Verification items for the finished model (mm, model axes). A direction names the side the tool comes from. Coordinates: 2 decimals unless noted, no trailing zeros. Order: outer loops, then holes, each group sorted by start corner. A loop starts at its lowest first (then second) coordinate and runs counter-clockwise, first axis right, second up. Notation, with made-up numbers: (57, 53.25) -> (102, 53.25) arc R17 cw to (102, 84.25) -> close; hole circle Ø9 at (84, 41). An arc over 180 degrees is marked (long way). Answer as CSV lines item,"result".
```python
from build123d import *

# Parameters (mm, degrees)
SKETCH_1_W          = 40
SKETCH_1_H          = 40
SKETCH_1_W_2        = 38
SKETCH_1_H_2        = 38
EXTRUDE_1_DEPTH     = 160
SKETCH_2_R          = 2.1
CUT_EXTRUDE_1_DEPTH = 170.705627485
SKETCH_4_R          = 2.1
CUT_EXTRUDE_2_DEPTH = 170.705627485


with BuildPart() as part:
    # 草图1 → 凸台-拉伸1 (new body)
    with BuildSketch(Plane.XY):
        with Locations((20, 20)):
            Rectangle(SKETCH_1_W, SKETCH_1_H)
        with Locations((20, 20)):
            Rectangle(SKETCH_1_W_2, SKETCH_1_H_2, mode=Mode.SUBTRACT)
    extrude(amount=EXTRUDE_1_DEPTH)

    # 草图2 → 切除-拉伸1 (cut, through all)
    with BuildSketch(Plane.XZ):
        with Locations(Location((8, 6, 0), (0, 0, 270))):
            Circle(SKETCH_2_R)
        with Locations(Location((32, 22, 0), (0, 0, 270))):
            Circle(SKETCH_2_R)
        with Locations(Location((8, 22, 0), (0, 0, 270))):
            Circle(SKETCH_2_R)
        with Locations(Location((32, 6, 0), (0, 0, 270))):
            Circle(SKETCH_2_R)
    extrude(amount=-CUT_EXTRUDE_1_DEPTH, mode=Mode.SUBTRACT)

    # 草图4 → 切除-拉伸2 (cut, through all)
    with BuildSketch(Plane.ZY):
        with Locations((138, 10)):
            Circle(SKETCH_4_R)
        with Locations((153, 30)):
            Circle(SKETCH_4_R)
        with Locations((153, 10)):
            Circle(SKETCH_4_R)
        with Locations((138, 30)):
            Circle(SKETCH_4_R)
        with Locations((83, 23)):
            Circle(SKETCH_4_R)
        with Locations((65, 7)):
            Circle(SKETCH_4_R)
        with Locations((65, 23)):
            Circle(SKETCH_4_R)
        with Locations((47, 7)):
            Circle(SKETCH_4_R)
        with Locations((47, 23)):
            Circle(SKETCH_4_R)
        with Locations((83, 7)):
            Circle(SKETCH_4_R)
    extrude(amount=-CUT_EXTRUDE_2_DEPTH, mode=Mode.SUBTRACT)


solid = part.part
```
Item 1: Tool access check on faces 4 (the cylindrical face through (39.49, 8.77, 48.13)), 5 (the flat face through (39, 20, 79)). Record the directions out of +Z, -Z, +X, -X, +Y, -Y that give a thin tool (end or side, any length) a straight path to the whole face; none if there is none.
Answer list:
face 4,"+X, -X"
face 5,"+Z, -Z"
Item 2: Section check D-D, the plane x = 32. Record the boundary of the cut face in (y, z).
Answer list:
outline,"(0, 0) -> (1, 0) -> (1, 3.9) -> (0, 3.9) -> close; (0, 8.1) -> (1, 8.1) -> (1, 19.9) -> (0, 19.9) -> close; (0, 24.1) -> (1, 24.1) -> (1, 160) -> (0, 160) -> close; (39, 0) -> (40, 0) -> (40, 3.9) -> (39, 3.9) -> close; (39, 8.1) -> (40, 8.1) -> (40, 19.9) -> (39, 19.9) -> close; (39, 24.1) -> (40, 24.1) -> (40, 160) -> (39, 160) -> close"
Item 3: Thickness scan on line 1 (Y direction, x = 0.5, z = 83); line 2 (X direction, y = 0.4, z = 6); line 3 (Y direction, x = 10.5, z = 144). Record the ranges inside material, lowest first.
Answer list:
line 1,"0 to 4.9, 9.1 to 20.9, 25.1 to 40"
line 2,"0 to 5.9, 10.1 to 29.9, 34.1 to 40"
line 3,"0 to 1, 39 to 40"
Item 4: Section check A-A, the plane z = 83. Record the boundary of the cut face in (x, y), plus the area to 3 significant figures.
Answer list:
outline,"(0, 0) -> (40, 0) -> (40, 4.9) -> (39, 4.9) -> (39, 1) -> (1, 1) -> (1, 4.9) -> (0, 4.9) -> close; (0, 9.1) -> (1, 9.1) -> (1, 20.9) -> (0, 20.9) -> close; (0, 25.1) -> (1, 25.1) -> (1, 39) -> (39, 39) -> (39, 25.1) -> (40, 25.1) -> (40, 40) -> (0, 40) -> close; (39, 9.1) -> (40, 9.1) -> (40, 20.9) -> (39, 20.9) -> close"
area,"139 mm2"
Item 5: Section check B-B, the plane y = 17. Record the boundary of the cut face in (x, z), plus the area to 3 significant figures.
Answer list:
outline,"(0, 0) -> (1, 0) -> (1, 160) -> (0, 160) -> close; (39, 0) -> (40, 0) -> (40, 160) -> (39, 160) -> close"
area,"320 mm2"
Item 6: Depth check by flat-ended pin: pin 1 Ø3.5 at (x, z) = (8, 6) entering from +Y. Enter the tip coordinate at first touch or a pass-through.
Answer list:
pin 1,"through"
Item 7: Release check for a two-part mould opening along Z. For faces 1 (the flat face through (20, 39, 79)), 2 (the flat face through (18.4, 0.8, 0)), 3 (the cylindrical face through (0.49, 7.09, 80.9)) record: +Z half, -Z half, draft (parallel to the pull), parting line (faces both ways), or undercut.
Answer list:
face 1,"draft"
face 2,"-Z half"
face 3,"undercut"
